```python
from build123d import *

# Parameters (mm, degrees)
BOSS_EXTRUDE1_DEPTH                    = 2.5
BOSS_EXTRUDE1_DEPTH_BACK               = 2.5
SKETCH1_W                              = 8
SKETCH1_H                              = 55
SKETCH2_R                              = 1.6
CUT_EXTRUDE1_DEPTH                     = 29.235615807
SKETCH3_W                              = 8
SKETCH3_H                              = 55
SKETCH3_R                              = 1.4
BOSS_EXTRUDE3_DEPTH                    = 5
CBORE_FOR_M5_HEX_HEAD_BOLT3_AT_2_COUNT = 2
CBORE_FOR_M5_HEX_HEAD_BOLT3_AT_2_PITCH = 22.5
CBORE_FOR_M5_HEX_HEAD_BOLT3_AT_3_COUNT = 2
CBORE_FOR_M5_HEX_HEAD_BOLT3_AT_3_PITCH = 45
CBORE_FOR_M5_HEX_HEAD_BOLT3_AT_4_COUNT = 2
CBORE_FOR_M5_HEX_HEAD_BOLT3_AT_4_PITCH = 22.5
FILLET1_R                              = 2


with BuildPart() as part:
    # Sketch1 → Boss-Extrude1 (new, two sides: drawn at the far end of the back side and taken through both)
    with BuildSketch(Plane.XY.offset(-BOSS_EXTRUDE1_DEPTH_BACK)):
        Rectangle(SKETCH1_W, SKETCH1_H)
    extrude(amount=BOSS_EXTRUDE1_DEPTH + BOSS_EXTRUDE1_DEPTH_BACK)

    # Sketch2 → Cut-Extrude1 (cut, through all)
    with BuildSketch(Plane.XY.offset(2.5)):
        with Locations((0, 22.5)):
            Circle(SKETCH2_R)
        with Locations((0, -22.5)):
            Circle(SKETCH2_R)
        Circle(SKETCH2_R)
    extrude(amount=-CUT_EXTRUDE1_DEPTH, mode=Mode.SUBTRACT)

    # Sketch3 → Boss-Extrude3 (add, through all)
    with BuildSketch(Plane.XY.offset(2.5)):
        with Locations((8, 0)):
            Rectangle(SKETCH3_W, SKETCH3_H)
        with Locations((8, 22.5)):
            Circle(SKETCH3_R, mode=Mode.SUBTRACT)
        with Locations((8, 0)):
            Circle(SKETCH3_R, mode=Mode.SUBTRACT)
        with Locations((8, -22.5)):
            Circle(SKETCH3_R, mode=Mode.SUBTRACT)
    extrude(amount=-BOSS_EXTRUDE3_DEPTH)

    # Sketch8 → CBORE for M5 Hex Head Bolt3 (revolve, cut)
    with BuildSketch(Plane(origin=(0, 22.5, -2.5), x_dir=(0, 1, 0), z_dir=(1, 0, 0))):
        Polygon((0, 0), (0, 5), (1.6, 5), (1.6, 3), (3.5, 3), (3.5, 0), align=None)
    cbore_for_m5_hex_head_bolt3 = revolve(axis=Axis((0, 22.5, -8.85), (0, 0, 1)), mode=Mode.SUBTRACT)

    # CBORE for M5 Hex Head Bolt3 at 2: CBORE for M5 Hex Head Bolt3 ×2
    with Locations(*[(0, -i * CBORE_FOR_M5_HEX_HEAD_BOLT3_AT_2_PITCH, 0) for i in range(1, CBORE_FOR_M5_HEX_HEAD_BOLT3_AT_2_COUNT)]):
        add(cbore_for_m5_hex_head_bolt3, mode=Mode.SUBTRACT)

    # CBORE for M5 Hex Head Bolt3 at 3: CBORE for M5 Hex Head Bolt3 ×2
    with Locations(*[(0, -i * CBORE_FOR_M5_HEX_HEAD_BOLT3_AT_3_PITCH, 0) for i in range(1, CBORE_FOR_M5_HEX_HEAD_BOLT3_AT_3_COUNT)]):
        add(cbore_for_m5_hex_head_bolt3, mode=Mode.SUBTRACT)

    # CBORE for M5 Hex Head Bolt3 at 4: CBORE for M5 Hex Head Bolt3 ×2
    with Locations(*[(0, -i * CBORE_FOR_M5_HEX_HEAD_BOLT3_AT_4_PITCH, 0) for i in range(1, CBORE_FOR_M5_HEX_HEAD_BOLT3_AT_4_COUNT)]):
        add(cbore_for_m5_hex_head_bolt3, mode=Mode.SUBTRACT)

    # Fillet1
    fillet1_edges = [part.edges().sort_by_distance(p)[0] for p in [
        (12, 27.5, 0),
        (12, -27.5, 0),
        (-4, -27.5, 0),
        (-4, 27.5, 0),
    ]]
    fillet(fillet1_edges, radius=FILLET1_R)


solid = part.part
```
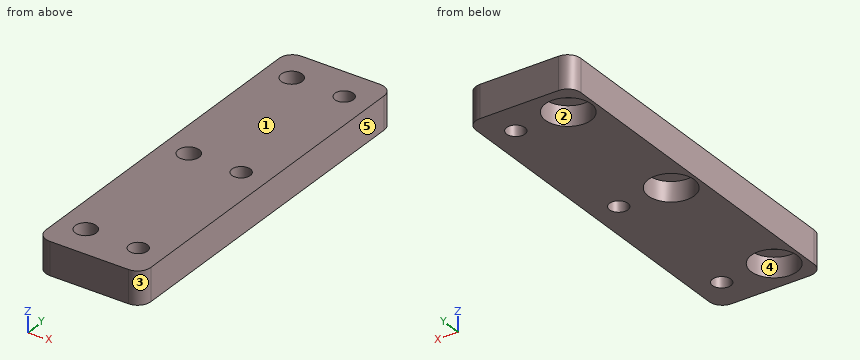
Build history of the part. All positions in model axes, mm. Face numbers are marked on the shaded views. A direction names the side the tool comes from. Round coordinates to 2 decimals unless told otherwise and drop trailing zeros. Order: outer loops, then holes, each group sorted by start corner. A loop starts at its lowest first (then second) coordinate and runs counter-clockwise, first axis right, second up. Notation, with made-up numbers: (3.25, 74) - (60.25, 74) arc R26 cw to (60.25, 109) - close; hole circle Ø6 at (19.25, -22.75). An arc over 180 degrees is marked (long way). Use a Markdown table: item, result.
1) Saw through at C-C on z = -0.3. Write the cut outline in (x, y), and give its area (3 significant figures).
Recorded:
| item | result |
|---|---|
| outline | (-4, -25.5) arc R2 ccw to (-2, -27.5) - (10, -27.5) arc R2 ccw to (12, -25.5) - (12, 25.5) arc R2 ccw to (10, 27.5) - (-2, 27.5) arc R2 ccw to (-4, 25.5) - close; hole circle Ø7 at (0, -22.5); hole circle Ø7 at (0, 0); hole circle Ø7 at (0, 22.5); hole circle Ø2.8 at (8, -22.5); hole circle Ø2.8 at (8, 0); hole circle Ø2.8 at (8, 22.5) |
| area | 743 mm² |
2) Wall check: L1, parallel to Y at x = 0, z = -1.05; L2, parallel to Y at x = 0, z = 1.7; L3, parallel to X at y = 0.5, z = -0.6. Give the ranges that are in metal, low to high.
Recorded:
| item | result |
|---|---|
| L1 | y = -27.5 to -26, -19 to -3.5, 3.5 to 19, 26 to 27.5 |
| L2 | y = -27.5 to -24.1, -20.9 to -1.6, 1.6 to 20.9, 24.1 to 27.5 |
| L3 | x = -4 to -3.46, 3.46 to 6.69, 9.31 to 12 |
3) Pull direction Y, two halves, no side cores. Call the marked faces 3, 4 and 5: pulls with the +Y half, pulls with the -Y half, needs draft (parallel to the pull), parting line crosses it, or undercut.
Recorded:
| item | result |
|---|---|
| face 3 | pulls with the -Y half |
| face 4 | undercut |
| face 5 | needs draft |
4) Saw through at B-B on x = 0. Write the cut outline in (y, z), and give its area (3 significant figures).
Recorded:
| item | result |
|---|---|
| outline | (-27.5, -2.5) - (-26, -2.5) - (-26, 0.5) - (-24.1, 0.5) - (-24.1, 2.5) - (-27.5, 2.5) - close; (-20.9, 0.5) - (-19, 0.5) - (-19, -2.5) - (-3.5, -2.5) - (-3.5, 0.5) - (-1.6, 0.5) - (-1.6, 2.5) - (-20.9, 2.5) - close; (1.6, 0.5) - (3.5, 0.5) - (3.5, -2.5) - (19, -2.5) - (19, 0.5) - (20.9, 0.5) - (20.9, 2.5) - (1.6, 2.5) - close; (24.1, 0.5) - (26, 0.5) - (26, -2.5) - (27.5, -2.5) - (27.5, 2.5) - (24.1, 2.5) - close |
| area | 193 mm² |
5) Flat gauge pins, fed straight in: pin 1 Ø2.5 at (x, y) = (0, -22.5) entering from +Z; pin 2 Ø4 at (x, y) = (0, 0) entering from -Z. Where does each tip first touch, or does it go through?
Recorded:
| item | result |
|---|---|
| pin 1 | passes through |
| pin 2 | stops at z = 0.5 |
6) Saw through at A-A on y = 0. Write the cut outline in (x, z).
Recorded:
| item | result |
|---|---|
| outline | (-4, -2.5) - (-3.5, -2.5) - (-3.5, 0.5) - (-1.6, 0.5) - (-1.6, 2.5) - (-4, 2.5) - close; (1.6, 0.5) - (3.5, 0.5) - (3.5, -2.5) - (6.6, -2.5) - (6.6, 2.5) - (1.6, 2.5) - close; (9.4, -2.5) - (12, -2.5) - (12, 2.5) - (9.4, 2.5) - close |
7) Tool access for the marked faces 1 and 2: list every direction of +Z, -Z, +X, -X, +Y, -Y with a clear straight run to the whole face (end or side of a thin tool).
Recorded:
| item | result |
|---|---|
| face 1 | +Z, +X, -X, +Y, -Y |
| face 2 | -Z |
